Geometry check sheet. Reference: the model listing, model coordinates, mm. A direction names the side the tool comes from. Round coordinates to 2 decimals unless told otherwise and drop trailing zeros. Order: outer loops, then holes, each group sorted by start corner. A loop starts at its lowest first (then second) coordinate and runs counter-clockwise, first axis right, second up. Notation, with made-up numbers: (47.5, 37) -> (57.5, 37) arc R5 ccw to (57.5, 45) -> close; hole circle Ø9 at (67.25, 89.5). An arc over 180 degrees is marked (long way). Answer as a JSON object with one key per item and string values. Group by question number.
from build123d import *

# Parameters (mm, degrees)
F0_R     = 36.5125
F1_DEPTH = 88.9
F2_R     = 19.05
F3_DEPTH = 88.901
F4_R     = 22.6187
F5_DEPTH = 15.9258


# Not quite as in the source:
# - a pattern or mirror of a feature is missing from the dataset's text; its kind, count and spacing are read off the source's solid


with BuildPart() as f1:
    # F0 (on Front) → F1 (new body)
    with BuildSketch(Plane.XZ):
        Circle(F0_R)
    extrude(amount=F1_DEPTH)

    # F2 (on Front) → F3 (cut, through all)
    with BuildSketch(Plane.XZ):
        Circle(F2_R)
    extrude(amount=F3_DEPTH, mode=Mode.SUBTRACT)

    # F4 (on Front) → F5 (cut)
    with BuildSketch(Plane.XZ):
        Circle(F4_R)
    f5 = extrude(amount=F5_DEPTH, mode=Mode.SUBTRACT)

    # F5_copies: F5 across plane
    add(f5.mirror(Plane(origin=(0, -44.45, 0), x_dir=(0, 0, -1), z_dir=(0, -1, 0))), mode=Mode.SUBTRACT)


solid = f1.part
Item 1: Sectioned sample at D-D, the plane x = -30. Enter the section's corners in (y, z).
Item 2: Sectioned sample at A-A, the plane x = 0. Enter the section's corners in (y, z).
Item 3: Set-up check for faces 1 (the cylindrical face through (21.574, -81.049, 6.794)), 2 (the cylindrical face through (34.826, -43.828, 10.967)), 3 (the flat face through (-12, -15.926, -15)): record each of +Z, -Z, +X, -X, +Y, -Y from which the full face is reachable in a straight line by a thin tool's end or side.
Item 4: Depth check by flat-ended pin: pin 1 Ø6 at (y, z) = (-59, 5) entering from +X; pin 2 Ø1.5 at (y, z) = (-29, 11) entering from +X; pin 3 Ø8 at (y, z) = (-14.5, -11) entering from +X. Enter the tip coordinate at first touch or a pass-through.
Item 5: Sectioned sample at B-B, the plane z = 0. Enter the section's corners in (x, y), then the cut area to 3 significant figures.
Item 6: Thickness scan on L1, parallel to Z at x = 0, y = -11.75; L2, parallel to X at y = -43, z = -0.5; L3, parallel to Z at x = 0, y = -39.5. Record the ranges inside material, lowest first.
Result:
{
 "1": {"outline": "(-88.9, -20.81) -> (0, -20.81) -> (0, 20.81) -> (-88.9, 20.81) -> close"},
 "2": {"outline": "(-88.9, -36.51) -> (0, -36.51) -> (0, -22.62) -> (-15.93, -22.62) -> (-15.93, -19.05) -> (-72.97, -19.05) -> (-72.97, -22.62) -> (-88.9, -22.62) -> close; (-88.9, 22.62) -> (-72.97, 22.62) -> (-72.97, 19.05) -> (-15.93, 19.05) -> (-15.93, 22.62) -> (0, 22.62) -> (0, 36.51) -> (-88.9, 36.51) -> close"},
 "3": {"face 1": "-Y", "face 2": "+Y, -Y", "face 3": "+Y"},
 "4": {"pin 1": "stops at x = 36.46", "pin 2": "stops at x = 35.04", "pin 3": "stops at x = 35.84"},
 "5": {"outline": "(-36.51, -88.9) -> (-22.62, -88.9) -> (-22.62, -72.97) -> (-19.05, -72.97) -> (-19.05, -15.93) -> (-22.62, -15.93) -> (-22.62, 0) -> (-36.51, 0) -> close; (19.05, -72.97) -> (22.62, -72.97) -> (22.62, -88.9) -> (36.51, -88.9) -> (36.51, 0) -> (22.62, 0) -> (22.62, -15.93) -> (19.05, -15.93) -> close", "area": "2,880 mm2"},
 "6": {"L1": "z = -36.51 to -22.62, 22.62 to 36.51", "L2": "x = -36.51 to -19.04, 19.04 to 36.51", "L3": "z = -36.51 to -19.05, 19.05 to 36.51"}
}
